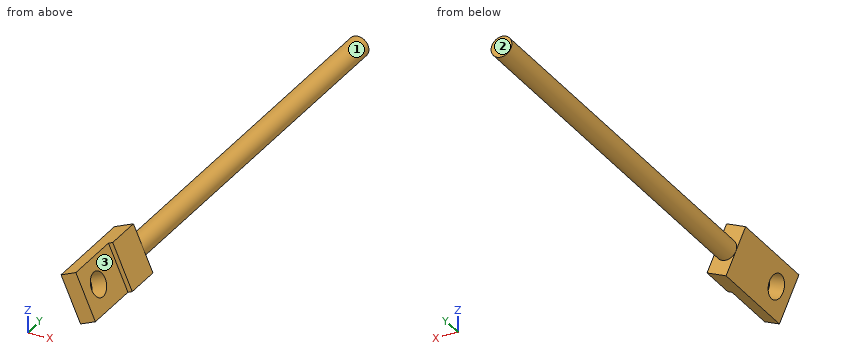
```python
from build123d import *

# Parameters (mm, degrees)
SKETCH2_R           = 3.5
BOSS_EXTRUDE1_DEPTH = 135
BOSS_EXTRUDE2_DEPTH = 7
SKETCH4_R           = 4
CUT_EXTRUDE1_DEPTH  = 7
SKETCH5_W           = 1.564160686
SKETCH5_H           = 19.573383476
CUT_EXTRUDE2_DEPTH  = 19.821098843


with BuildPart() as part:
    # Sketch2 → Boss-Extrude1 (new body)
    with BuildSketch(Plane(origin=(0, 0, 0), x_dir=(1, 0, 0), z_dir=(0, 1, 0))):
        with Locations((-10.295474734, 5.826559877)):
            Circle(SKETCH2_R)
    extrude(amount=BOSS_EXTRUDE1_DEPTH)

    # Sketch3 → Boss-Extrude2 (add)
    with BuildSketch(Plane(origin=(-7.567781688, 0, -3.338011531), x_dir=(-0.403567776, 0, 0.914949753), z_dir=(-0.914949753, 0, -0.403567776))):
        Polygon((-9.296087677, 0.018668346), (-9.296087677, -32), (6.940301507, -32), (6.940301507, 0), align=None)
    extrude(amount=BOSS_EXTRUDE2_DEPTH)

    # Sketch4 → Cut-Extrude1 (cut)
    with BuildSketch(Plane(origin=(-7.567781688, 0, -3.338011531), x_dir=(0.403567776, 0, -0.914949753), z_dir=(0.914949753, 0, 0.403567776))):
        with Locations((0.894610349, -24.070410288)):
            Circle(SKETCH4_R)
    extrude(amount=-CUT_EXTRUDE1_DEPTH, mode=Mode.SUBTRACT)

    # Sketch5 → Cut-Extrude2 (cut, through all)
    with BuildSketch(Plane(origin=(-2.800882044, 0, 6.350027148), x_dir=(0.914949753, 0, 0.403567776), z_dir=(-0.403567776, 0, 0.914949753))):
        with Locations((-9.053334217, -22.213308262)):
            Rectangle(SKETCH5_W, SKETCH5_H)
    extrude(amount=-CUT_EXTRUDE2_DEPTH, mode=Mode.SUBTRACT)


solid = part.part
```
Could you check a few things on this model? Use its own coordinates, in mm. Face numbers are marked on the shaded views. A direction names the side the tool comes from. Round coordinates to 2 decimals unless told otherwise and drop trailing zeros. Write each loop counter-clockwise with the first axis right and the second up, starting at its lowest first coordinate (ties: lowest second). Pieces come first, ordered by that corner, then holes.
(1) For pin 1 (4 mm diameter, centred on x = -14, y = -6.5, fed in from +Z); pin 2 (3 mm diameter, centred on x = -12, z = -10, fed in from +Y); pin 3 (6 mm diameter, centred on y = 53, z = -5, fed in from -X); pin 4 (4 mm diameter, centred on x = -6, z = -4.5, fed in from -Y), each with a flat end and sliding along its axis, tell me the tip position at first contact or that it passes through.
Findings below:
pin 1: stops at z = 2.29
pin 2: stops at y = 135
pin 3: stops at x = -13.8
pin 4: stops at y = -12.43
(2) Which directions (+Z, -Z, +X, -X, +Y, -Y) give clear straight access to the entire face, cutting with the end or side of a thin tool? Please do the marked faces 1, 2 and 3.
Findings below:
face 1: +Y
face 2: +Z, -Z, +X, -X, +Y
face 3: +Z, +X, -Y
(3) If I drill on probe 1 along Y at (x, z) = (-11, -3.75); probe 2 along Y at (x, z) = (-11, 0.25); probe 3 along Y at (x, z) = (-5.25, -10), over which ranges is the centre line in solid material (lowest first)?
Findings below:
probe 1: y = -32 to -27.59, -20.55 to 135
probe 2: y = -32 to 0
probe 3: y = -12.43 to 0.02
(4) Suppose I cut it at A-A on y = 51. Write out the boundary of the cut face in (x, z), and give its area (3 significant figures).
Findings below:
outline: circle Ø7 at (-10.3, -5.83)
area: 38.5 mm2
